Autodesk Inventor part; units mm, degrees
ref_plane "Work Plane1" through (0, 0, 0) normal (0, 0, 1) x (1, 0, 0)
ref_plane "YZ Plane" through (0, 0, 0) normal (1, 0, 0) x (0, 1, 0)
ref_plane "XZ Plane" through (0, 0, 0) normal (0, 1, 0) x (-1, 0, 0)
ref_plane "Work Plane1" through (0, 0, 0) normal (0, 0, 1) x (1, 0, 0)
sketch "Sketch1" plane through (0, 0, 0) normal (0, 0, 1) x (1, 0, 0)
  circle A0 centre (-83.6503, 950) radius 2.1
  circle A1 centre (-83.6503, 970) radius 2.1
  circle A2 centre (-63.6503, 950) radius 2.1
  circle A3 centre (-43.6503, 950) radius 2.1
  circle A4 centre (-23.6503, 950) radius 2.1
  circle A5 centre (-23.6503, 970) radius 2.1
  line L0 (-3.55, 0) -> (-3.55, 1000)
  line L1 (16.25, 0) -> (16.25, 1000)
  line L2 (-58.7503, 960) -> (-48.5503, 960)
  line L3 (-73.6503, 979.5) -> (-73.6503, 974.8314)
  line L4 (-78.7503, 980) -> (-74.1503, 980)
  line L5 (-33.6503, 974.8314) -> (-33.6503, 979.5)
  line L6 (-33.1503, 980) -> (-28.5503, 980)
  line L7 (-33.6503, 960) -> (-33.6503, 965.1685)
  line L8 (-38.7503, 960) -> (-33.6503, 960)
  line L9 (-73.6503, 960) -> (-68.5503, 960)
  line L10 (-73.6503, 965.1685) -> (-73.6503, 960)
  line L11 (-93.1503, 980) -> (-88.5503, 980)
  line L12 (-93.6503, 974.8314) -> (-93.6503, 979.5)
  line L13 (-93.6503, 960.207) -> (-93.6386, 965.287)
  line L14 (-93.6503, 954.8314) -> (-93.6503, 959.793)
  line L15 (-93.6503, 940.5) -> (-93.6503, 945.1685)
  line L16 (-88.4817, 940) -> (-93.1503, 940)
  line L17 (-14.1503, 940) -> (-18.8188, 940)
  circle A6 centre (-3.55, 950) radius 2.55
  circle A7 centre (16.25, 950) radius 2.55
  line L18 (26.35, 0) -> (26.35, 1000)
  line L19 (-14.1503, 940) -> (26.35, 940)
  line L20 (-14.1503, 940) -> (-93.1503, 940)
  line L21 (-33.6503, 960) -> (-33.7332, 960)
  line L22 (-14.15, 1000) -> (26.35, 1000)
  line L23 (26.35, 940) -> (26.35, 1000)
  line L24 (-33.6503, 960) -> (-33.6503, 960.1732)
  line L25 (-93.1503, 940) -> (-93.6503, 940)
  line L26 (-93.6503, 940) -> (-93.6503, 980)
  line L27 (-93.6503, 980) -> (-93.1503, 980)
  line L28 (-93.6503, 950) -> (27.9251, 950) construction
  circle A8 centre (-3.55, 985) radius 2.55
  circle A9 centre (16.25, 985) radius 2.55
  circle A10 centre (-80.3911, 959.775) radius 2.5
  circle A11 centre (-74.1633, 1006.5119) radius 2.5
  circle A12 centre (-33.6542, 953.5473) radius 2.5
  line L29 (-85.3287, 955.7671) -> (-21.9733, 1004.2234) construction
  line L30 (-29.4228, 948.3176) -> (-77.6558, 1011.3809) construction
  line L31 (-24.4599, 1000) -> (-14.15, 1000)
  line L32 (-93.6503, 980) -> (-93.6503, 1018.8249)
  line L33 (-93.6503, 1018.8249) -> (-53.65, 1018.8249)
  line L34 (-24.4599, 1000) -> (-53.65, 1018.8249)
  line L35 (-53.6502, 925.444) -> (-53.6503, 1034.9111) construction
  line L36 (-107.7091, 987) -> (-12.8224, 987) construction
  line L37 (-76.4503, 980) -> (8.1353, 980) construction
  line L38 (-33.6542, 953.5473) -> (-80.3911, 959.775) construction
  circle A13 centre (-53.6503, 980) radius 11.05
  circle A14 centre (-83.6503, 970) radius 2.55
  circle A15 centre (-83.6503, 950) radius 2.55
  circle A16 centre (-23.6503, 950) radius 2.55
  circle A17 centre (-63.6503, 950) radius 2.55
  circle A18 centre (-23.6503, 970) radius 2.55
  point P0 (0, 0)
  point P1 (-53.65, 970.886)
  point P2 (-93.65, 979.5)
  point P3 (-93.65, 974.8315)
  point P4 (-93.65, 959.793)
  point P5 (-93.65, 954.8315)
  point P6 (-93.65, 945.1686)
  point P7 (-93.65, 940.5)
  point P8 (-88.4815, 940)
  point P9 (-18.8186, 940)
  point P10 (-88.4816, 940)
  dimension "d0" = 5.1
  dimension "d2" = 5.1
  dimension "d9" = 5.1
  dimension "d10" = 15
  dimension "d11" = 15
  dimension "d17" = 47.15
  dimension "d22" = 5
  dimension "d23" = 5
  dimension "d24" = 5
  dimension "d29" = 20
  dimension "d30" = 7
  dimension "d31" = 47.15
  dimension "d32" = 22.1
  dimension "d33" = 5.1
  dimension "d34" = 5.1
  dimension "d35" = 5.1
  dimension "d36" = 5.1
  dimension "d37" = 5.1
extrude "Extrusion1" add sketch "Sketch1" along normal blind 5 contours A0 | A1 | A2 | A3 | A4 | A5 | L19 L17 L20 L16 L25 L26 L15 L14 L12 L32 L33 L34 L31 L22 L0 A8 A6 | L0 A6 A8 L22 L1 A9 A7 L19 | A6 L0 | L0 A6 | L1 A7 A9 L22 L18 L19 | A7 L1 | L1 A7 | A8 L0 | L0 A8 | A9 L1 | L1 A9 | A10 | A11 | A12 | A13 | A14 | A15 | A16 | A17 | A18
sketch "Sketch6" plane through (0, 0, 0) normal (0, 0, -1) x (-1, 0, 0)
  point P0 (0, 0)
  point P1 (83.6421, 950.0283)
  point P2 (63.6777, 949.9996)
  point P3 (23.6294, 949.9891)
  point P4 (3.544, 949.9934)
  point P5 (-16.2696, 949.986)
  point P6 (-16.2577, 984.9913)
  point P7 (3.5466, 984.9939)
  point P8 (74.1659, 1006.5019)
  point P9 (83.651, 970.0009)
  point P10 (80.4004, 959.774)
  point P11 (33.6669, 953.5674)
  point P12 (23.6003, 970.0426)
hole "Hole3" at (-83.6421, 950.0283, 0) at (-63.6777, 949.9996, 0) at (-23.6294, 949.9891, 0) at (-3.544, 949.9934, 0) at (16.2696, 949.986, 0) at (16.2577, 984.9913, 0) at (-3.5466, 984.9939, 0) at (-74.1659, 1006.5019, 0) at (-83.651, 970.0009, 0) at (-80.4004, 959.774, 0) at (-33.6669, 953.5674, 0) at (-23.6003, 970.0426, 0) direction (0, 0, 1) diameter 5.1 end through all
sketch "Sketch7" plane through (0, 0, 5) normal (0, 0, -1) x (-1, 0, 0)
  circle A0 centre (53.6503, 979) radius 4
  circle A1 centre (53.6503, 979) radius 11.25
  point P0 (0, 0)
  dimension "d59" = 22.5
extrude "Extrusion2" cut sketch "Sketch7" along normal blind 5 contours A0 | A1
properties part number "Y axis motor mount_3DPrint"
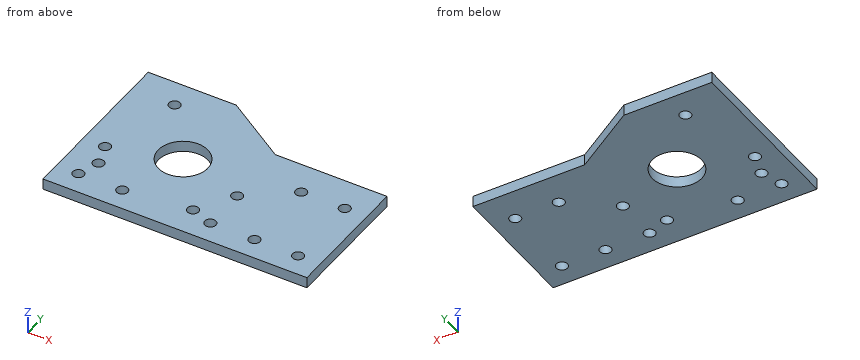
Geometry check sheet. Reference: the model listing, model coordinates, mm. Round coordinates to 2 decimals unless told otherwise and drop trailing zeros. Order: outer loops, then holes, each group sorted by start corner. A loop starts at its lowest first (then second) coordinate and runs counter-clockwise, first axis right, second up. Notation, with made-up numbers: M -33,13 L 16,13 A15 cw 16,17 Z; hole C -36.75,-21 d8. An arc over 180 degrees is marked long. Write each question's results on one line, items separated by ' | '. Start each with the question number.
1. Go/stop test with flat-tipped pins: P1, Ø1.5, axis at x = 1.5, z = 2.5, coming from the +Y side; P2, Ø3, axis at x = -83.64, y = 950.03, coming from the +Z side. Record where each tip stops, or that it passes through.
2. Cross-section at D-D on x = -9. Record the boundary of the cut face in (y, z).
3. Material ranges on L1, parallel to Y at x = -83.5, z = 4.55; L2, parallel to Y at x = -76, z = 0.5; L3, parallel to Y at x = 12, z = 3.2, recorded low to high. Write a range as from..to.
4. Cross-section at A-A on y = 979. Record the boundary of the cut face in (x, z).
5. Cross-section at B-B on z = 1.75. Give the number of separate pieces and of enclosed holes in the cut face, plus the area to 3 significant figures.
6. Cross-section at C-C on x = -52. Record the boundary of the cut face in (y, z).
Resolved:
1) P1: y = 1000 | P2: through
2) outline: M 940,0 L 1000,0 L 1000,5 L 940,5 Z
3) L1: 940..947.48, 952.57..967.46, 972.55..1018.82 | L2: 940..1004.73, 1008.27..1018.82 | L3: 940..1000
4) outline: M -93.65,0 L -64.9,0 L -64.9,5 L -93.65,5 Z; M -42.4,0 L 26.35,0 L 26.35,5 L -42.4,5 Z
5) separate pieces: 1 | enclosed holes: 13 | area: 7,590 mm2
6) outline: M 940,0 L 967.87,0 L 967.87,5 L 940,5 Z; M 990.13,0 L 1017.76,0 L 1017.76,5 L 990.13,5 Z
